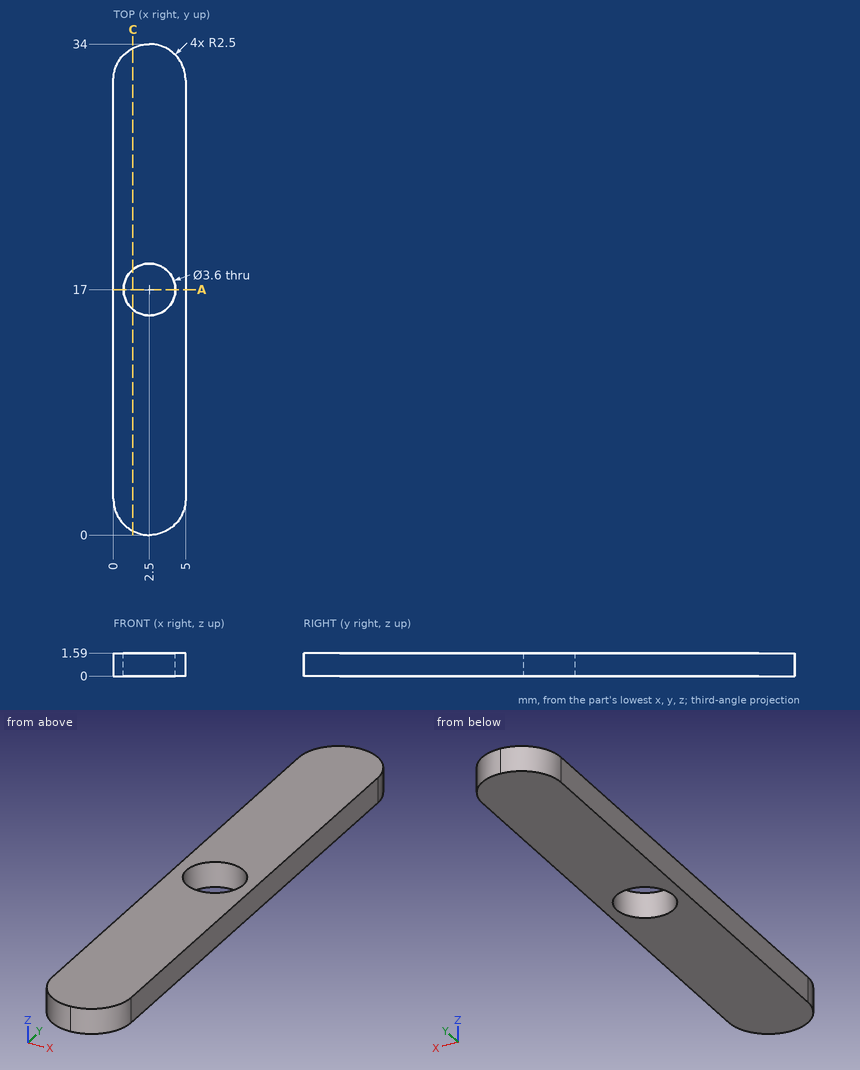
Input: dimensioned drawing with shaded views. Units: mm. Origin: part minimum x, y, z. Round coordinates to 2 decimals unless told otherwise and drop trailing zeros. Loops run counter-clockwise (first coordinate to the right, second up) from the corner with the lowest first, then second, coordinate; pieces in that order, holes last. Notation, with made-up numbers: (54.25, 47.25) -> (69.25, 47.25) arc R14 cw to (69.25, 65.25) -> close; hole circle Ø8 at (9.5, 22.5). An arc over 180 degrees is marked (long way). Use one line per item in the form item = value. Start each with the question number.
1) Section C-C on x = 1.35. Output: boundary loops of the cut face in (y, z) (1 decimal).
2) Section A-A on y = 17. Output: boundary loops of the cut face in (x, z).
3) Line query: L1, parallel to Y at x = 2.5, z = 0.7; L2, parallel to X at y = 17, z = 1.15; L3, parallel to Y at x = 3.6, z = 0.15 (1 decimal). Output: solid intervals per line, ascending.
Response:
q1.outline = (0.3, 0) -> (15.6, 0) -> (15.6, 1.6) -> (0.3, 1.6) -> close; (18.4, 0) -> (33.7, 0) -> (33.7, 1.6) -> (18.4, 1.6) -> close
q2.outline = (0, 0) -> (0.7, 0) -> (0.7, 1.59) -> (0, 1.59) -> close; (4.3, 0) -> (5, 0) -> (5, 1.59) -> (4.3, 1.59) -> close
q3.L1 = 0 to 15.2, 18.8 to 34
q3.L2 = 0 to 0.7, 4.3 to 5
q3.L3 = 0.3 to 15.6, 18.4 to 33.7
